For this review, take the finished solid that the model builds, in its own axes (mm). Face numbers are marked on the shaded views. A direction names the side the tool comes from. Coordinates: 2 decimals unless noted, no trailing zeros. Loops run counter-clockwise (first coordinate to the right, second up) from the corner with the lowest first, then second, coordinate; pieces in that order, holes last. Notation, with made-up numbers: M 0.25,0.25 L 37.25,0.25 A20 cw 37.25,7.25 Z; hole C 48.5,26.25 d11. An arc over 180 degrees is marked long. Answer as a JSON object with one key per item and string values. Group by question number.
Item 1: Tool access review of the marked faces 1, 2 and 3: name each direction out of +Z, -Z, +X, -X, +Y, -Y from which nothing blocks a thin tool from reaching the whole face with its end or side.
Item 2: Add section D-D (y = 1.5). State the section outline as (x, z) points.
Item 3: Wall thickness on L1, parallel to Z at x = 27.5, y = 0.75; L2, parallel to X at y = 5.25, z = -6.5; L3, parallel to Z at x = -1.5, y = 6.5: over which ranges is each line inside the solid? List them lowest first. Write a range as from..to.
Item 4: Add section B-B (x = 64.75). State the section outline as (y, z) points, then the cut area to 3 significant figures.
Item 5: Add section C-C (x = 36.5). State the section outline as (y, z) points.
Item 6: Add section A-A (z = -32). State the section outline as (x, y) points.
Item 7: Mouldability with a two-part tool opening along X and no side actions: class the marked faces 4, 5 and 6 as +X half, -X half, draft (parallel to the pull), parting line (faces both ways), or undercut.
Item 8: Insertion check: pin 1 (7 mm diameter, centred on y = 5.5, z = -41, fed in from +X); pin 2 (1 mm diameter, centred on x = 13.5, z = -44.5, fed in from +Y); pin 3 (3 mm diameter, centred on x = 29.5, y = 12, fed in from -Z). Each pin has a flat end and moves straight along its axis. Give the tip position at first contact, or say it passes through.
from build123d import *

# Parameters (mm, degrees)
BOSS_EXTRUDE1_DEPTH = 13.6
BOSS_EXTRUDE2_DEPTH = 3
FILLET1_START       = -66.6
FILLET1_DEPTH       = 71.6
FILLET1_START_2     = -6
FILLET1_2_DEPTH     = 69
SKETCH3_W           = 6
SKETCH3_H           = 71.6
BOSS_EXTRUDE4_DEPTH = 3


with BuildPart() as part:
    # Sketch1 → Boss-Extrude1 (new body)
    with BuildSketch(Plane(origin=(0, 0, 0), x_dir=(1, 0, 0), z_dir=(0, 1, 0))):
        Polygon((56.75, 30.8), (61.75, 30.8), (61.75, 66.6), (-5, 66.6), (-5, 33.8), (0, 33.8), (0, 61.6), (56.75, 61.6), align=None)
        Polygon((-5, 27.8), (-5, -5), (61.75, -5), (61.75, 30.8), (56.75, 30.8), (56.75, 0), (0, 0), (0, 27.8), align=None)
    extrude(amount=BOSS_EXTRUDE1_DEPTH)

    # Sketch2 → Boss-Extrude2 (add)
    with BuildSketch(Plane.XZ):
        Polygon((0, 0), (56.75, 0), (56.75, -61.6), (0, -61.6), (0, -33.8), (-5, -33.8), (-5, -66.6), (61.75, -66.6), (61.75, 5), (-5, 5), (-5, -27.8), (0, -27.8), align=None)
        Polygon((-5, -27.8), (-5, -33.8), (0, -33.8), (0, -61.6), (56.75, -61.6), (56.75, 0), (0, 0), (0, -27.8), align=None)
    extrude(amount=BOSS_EXTRUDE2_DEPTH)

    # Fillet1: read off the stored shape, not the designer's step
    # Fillet1 outline → Fillet1 (cut)
    with BuildSketch(Plane.XY.offset(FILLET1_START)):
        with BuildLine():
            Line((-5, 13.6), (-5, 8.6))
            ThreePointArc((-5, 8.6), (-3.535533906, 12.135533906), (0, 13.6))
            Line((0, 13.6), (-5, 13.6))
        make_face()
        with BuildLine():
            Line((61.75, 13.6), (56.75, 13.6))
            ThreePointArc((56.75, 13.6), (60.285533906, 12.135533906), (61.75, 8.6))
            Line((61.75, 8.6), (61.75, 13.6))
        make_face()
    extrude(amount=FILLET1_DEPTH, mode=Mode.SUBTRACT)

    # Fillet1 2 outline → Fillet1 2 (cut)
    with BuildSketch(Plane.YZ.offset(FILLET1_START_2)):
        with BuildLine():
            Line((13.6, 5), (8.6, 5))
            ThreePointArc((8.6, 5), (12.135533906, 3.535533906), (13.6, 0))
            Line((13.6, 0), (13.6, 5))
        make_face()
        with BuildLine():
            ThreePointArc((13.6, -61.6), (12.135533906, -65.135533906), (8.6, -66.6))
            Line((8.6, -66.6), (13.6, -66.6))
            Line((13.6, -66.6), (13.6, -61.6))
        make_face()
    extrude(amount=FILLET1_2_DEPTH, mode=Mode.SUBTRACT)

    # Sketch3 → Boss-Extrude4 (add)
    with BuildSketch(Plane.XZ.offset(3)):
        with Locations((64.75, -30.8)):
            Rectangle(SKETCH3_W, SKETCH3_H)
        with BuildLine():
            ThreePointArc((62.9, -62.6), (64.75, -64.45), (66.6, -62.6))
            Line((66.6, -62.6), (66.6, 1))
            ThreePointArc((66.6, 1), (64.75, 2.85), (62.9, 1))
            Line((62.9, 1), (62.9, -62.6))
        make_face(mode=Mode.SUBTRACT)
    extrude(amount=-BOSS_EXTRUDE4_DEPTH)


solid = part.part
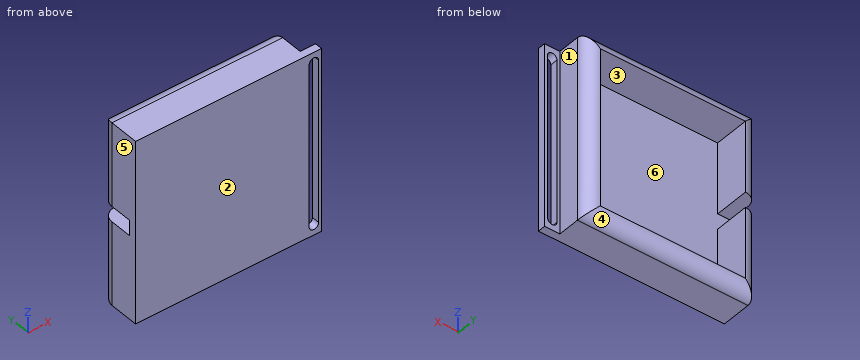
From the geometry:
{
 "1": {"face 1": "+Z, -Z, +X, +Y", "face 2": "+Z, -Z, +X, -X, -Y", "face 3": "+Y"},
 "2": {"outline": "M -5,-66.6 L 61.75,-66.6 L 61.75,5 L -5,5 L -5,-27.8 L 0,-27.8 L 0,0 L 56.75,0 L 56.75,-61.6 L 0,-61.6 L 0,-33.8 L -5,-33.8 Z"},
 "3": {"L1": "z = -66.6..-61.6, 0..5", "L2": "x = -5..0, 56.75..61.75", "L3": "z = -66.6..-33.8, -27.8..5"},
 "4": {"outline": "M -3,-66.6 L 0,-66.6 L 0,-64.45 L -3,-64.45 Z; M -3,2.85 L 0,2.85 L 0,5 L -3,5 Z", "area": "12.9 mm²"},
 "5": {"outline": "M -3,-66.6 L 8.6,-66.6 A5 ccw 13.6,-61.6 L 0,-61.6 L 0,0 L 13.6,0 A5 ccw 8.6,5 L -3,5 Z"},
 "6": {"outline": "M -5,-3 L 62.9,-3 L 62.9,0 L 61.75,0 L 61.75,8.6 A5 ccw 56.75,13.6 L 56.75,0 L -5,0 Z; M 66.6,-3 L 67.75,-3 L 67.75,0 L 66.6,0 Z"},
 "7": {"face 4": "draft", "face 5": "-X half", "face 6": "undercut"},
 "8": {"pin 1": "stops at x = 61.75", "pin 2": "stops at y = 0", "pin 3": "stops at z = -66.22"}
}
